Model file for the job. Use its own axes, mm. Round coordinates to 2 decimals unless told otherwise and drop trailing zeros. Loops run counter-clockwise (first coordinate to the right, second up) from the corner with the lowest first, then second, coordinate; pieces in that order, holes last. Notation, with made-up numbers: M 8.25,-19.5 L 59.25,-19.5 A33 cw 59.25,14.5 Z; hole C -33,0.25 d6. An arc over 180 degrees is marked long. Use a Markdown table: item, result. Add a question column.
Q1. Cut at B-B (z = 3.25). Give the cut face in (x, y), plus the area to 3 significant figures.
Q2. Cut at A-A (y = -9.75). Give the cut face in (x, z).
Q3. Pin check, flat tip, straight feed: pin 1 (2 mm diameter, centred on x = 8.5, z = -10, fed in from +Y). Stop position of the tip, or through.
Q4. Probe line 1 (X direction, y = 7.75, z = -4.25); line 2 (X direction, y = -0.25, z = 7.75); line 3 (Y direction, x = 8, z = -7.75). List the from-to ranges inside material, lowest first. Write a range as from..to.
from build123d import *

# Parameters (mm, degrees)
F0_W     = 25.4
F0_H     = 25.4
F1_DEPTH = 12.7
F2_SIZE  = 5.08
F3_R     = 5.08


with BuildPart() as f1:
    # F0 (on Front) → F1 (new body, symmetric)
    with BuildSketch(Plane.XZ):
        Rectangle(F0_W, F0_H)
    extrude(amount=F1_DEPTH, both=True)

    # F2
    f2_edges = [f1.edges().sort_by_distance(p)[0] for p in [
        (0, -12.7, 12.7),
        (-12.7, 0, 12.7),
        (-12.7, -12.7, 0),
    ]]
    chamfer(f2_edges, length=F2_SIZE)

    # F3
    f3_edges = [f1.edges().sort_by_distance(p)[0] for p in [
        (12.7, 12.7, 0),
        (12.7, 0, -12.7),
        (0, 12.7, -12.7),
    ]]
    fillet(f3_edges, radius=F3_R)


solid = f1.part
Checked values:
| question | item | result |
|---|---|---|
| 1 | outline | M -12.7,-7.62 L -7.62,-12.7 L 12.7,-12.7 L 12.7,7.62 A5.08 ccw 7.62,12.7 L -12.7,12.7 Z |
| 1 | area | 627 mm^2 |
| 2 | outline | M -10.57,-12.7 L 7.62,-12.7 A5.08 ccw 12.7,-7.62 L 12.7,10.57 L -7.62,10.57 L -10.57,7.62 Z |
| 3 | pin 1 | stops at y = 12.46 |
| 4 | line 1 | x = -12.7..12.7 |
| 4 | line 2 | x = -12.57..12.7 |
| 4 | line 3 | y = -12.7..12.68 |
